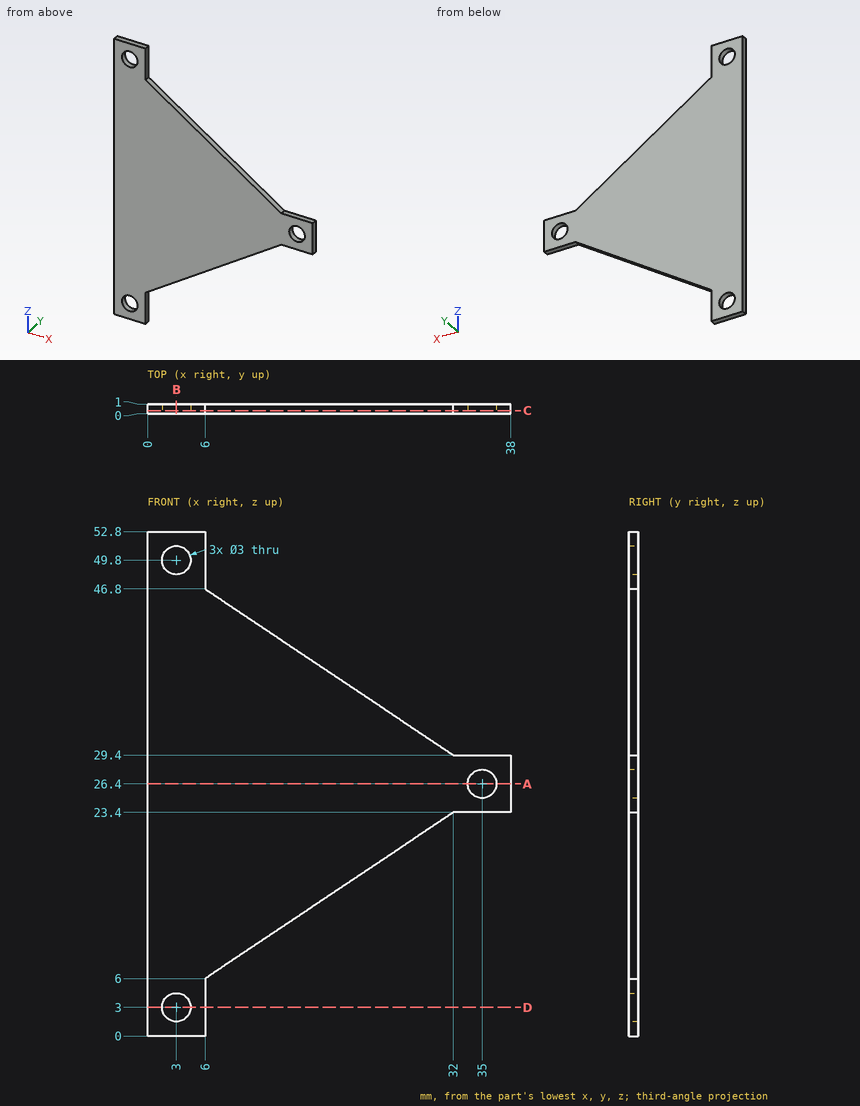
Study the drawing (mm; zero at the part's minimum x, y, z) and answer. Give positions to 0.01 mm unless a question says otherwise; leave off trailing zeros. Order: outer loops, then holes, each group sorted by start corner. A loop starts at its lowest first (then second) coordinate and runs counter-clockwise, first axis right, second up. Notation, with made-up numbers: (84, -16.75) - (107, -16.75) arc R15 ccw to (107, 10.25) - close; hole circle Ø3 at (-22.75, 39). An arc over 180 degrees is marked (long way). Answer in a Markdown table with one row per item. Add a question column.
Q1. The part is cut by section A-A (z = 26.4). Determine the outline of the cut face in (x, y), then the cut area to 3 significant figures.
Q2. The part is cut by section C-C (y = 0.3). Determine the outline of the cut face in (x, z).
Q3. Given P1, Ø12, axis at x = 32, z = 11, coming from the -Y side; P2, Ø0.5, axis at x = 36, y = 0.5, coming from the -Z side, each flat-ended and moving along its own axis, determine where each tip first touches the part or whether it passes through.
Q4. Find the intervals of material crossed by line 1 along X through (y, z) = (0.25, 26.4); line 2 along X through (y, z) = (0.35, 3); line 3 along Z through (x, y) = (2, 0.85), in increasing order. Write a range as [from, to].
Q5. The part is cut by section B-B (x = 3). Determine the outline of the cut face in (y, z).
Q6. The part is cut by section D-D (z = 3). Determine the outline of the cut face in (x, y), then the cut area to 3 significant figures.
Determined:
| question | item | result |
|---|---|---|
| 1 | outline | (0, 0) - (33.5, 0) - (33.5, 1) - (0, 1) - close; (36.5, 0) - (38, 0) - (38, 1) - (36.5, 1) - close |
| 1 | area | 35.0 mm² |
| 2 | outline | (0, 0) - (6, 0) - (6, 6) - (32, 23.4) - (38, 23.4) - (38, 29.4) - (32, 29.4) - (6, 46.8) - (6, 52.8) - (0, 52.8) - close; hole circle Ø3 at (3, 3); hole circle Ø3 at (3, 49.8); hole circle Ø3 at (35, 26.4) |
| 3 | P1 | passes through |
| 3 | P2 | stops at z = 23.4 |
| 4 | line 1 | x = [0, 33.5], [36.5, 38] |
| 4 | line 2 | x = [0, 1.5], [4.5, 6] |
| 4 | line 3 | z = [0, 1.88], [4.12, 48.68], [50.92, 52.8] |
| 5 | outline | (0, 0) - (1, 0) - (1, 1.5) - (0, 1.5) - close; (0, 4.5) - (1, 4.5) - (1, 48.3) - (0, 48.3) - close; (0, 51.3) - (1, 51.3) - (1, 52.8) - (0, 52.8) - close |
| 6 | outline | (0, 0) - (1.5, 0) - (1.5, 1) - (0, 1) - close; (4.5, 0) - (6, 0) - (6, 1) - (4.5, 1) - close |
| 6 | area | 3.00 mm² |
